Input: dimensioned drawing with shaded views. Units: mm. Origin: part minimum x, y, z. Round coordinates to 2 decimals unless told otherwise and drop trailing zeros. Write each loop counter-clockwise with the first axis right and the second up, starting at its lowest first coordinate (ties: lowest second). Pieces come first, ordered by that corner, then holes. Notation, with made-up numbers: (33.5, 19) - (68.5, 19) arc R7 ccw to (68.5, 24) - close; hole circle Ø8 at (66, 82.5). An arc over 180 degrees is marked (long way). Write item = value, one per line. Start each with the question number.
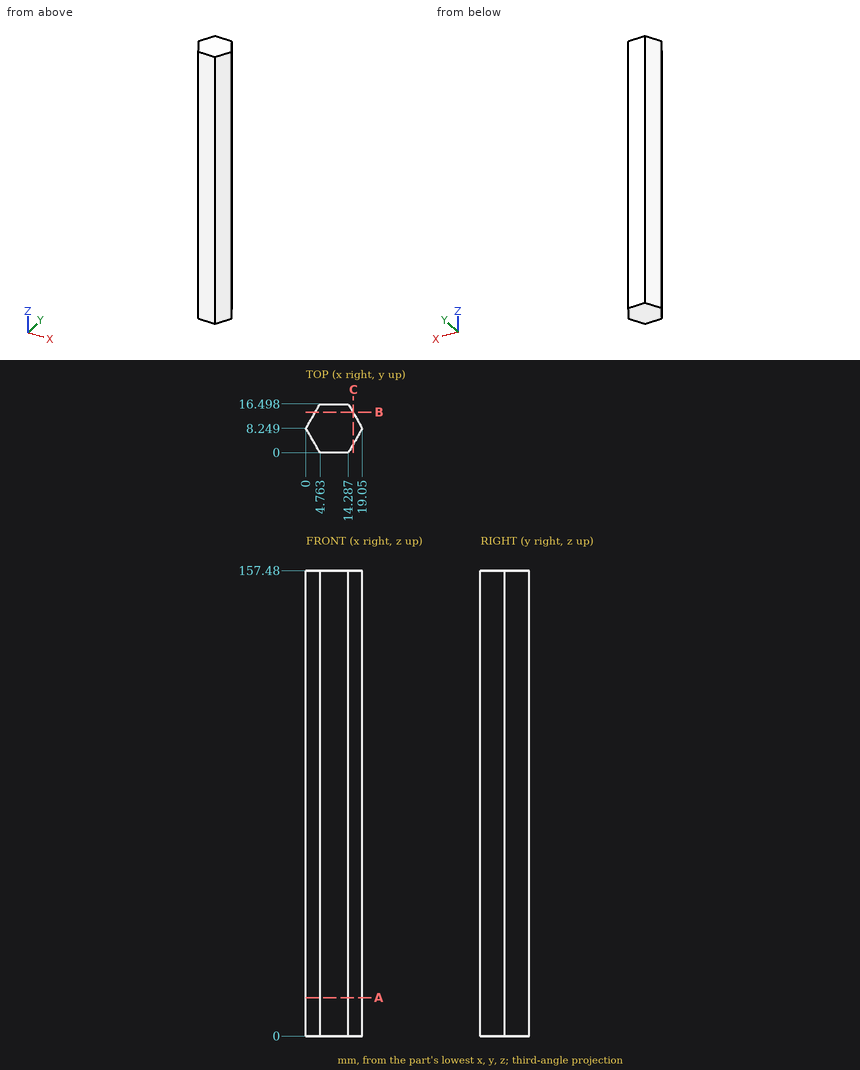
(1) Contact query for flat-ended pins moving along their axis: P1, Ø1.5, axis at y = 4, z = 103, coming from the +X side; P2, Ø1, axis at y = 10, z = 130, coming from the +X side; P3, Ø2, axis at x = 3.5, z = 86, coming from the -Y side (1 decimal). Output: stop coordinate, or through.
(2) Ray query, L1, parallel to Y at x = 4.75, z = 53.5 (1 decimal); L2, parallel to X at y = 14.5, z = 126; L3, parallel to X at y = 7, z = 48.5. Return the intervals inside material, ascending. Write a range as from..to.
(3) Section B-B (y = 13.75). Return the cut outline in (x, z).
(4) Section C-C (x = 16). Return the cut outline in (y, z), plus the area to 3 significant figures.
(5) Section A-A (z = 13). Return the cut outline in (x, y).
Solution:
q1.P1 = 17.03
q1.P2 = 18.33
q1.P3 = 0.5
q2.L1 = 0..16.5
q2.L2 = 3.61..15.44
q2.L3 = 0.72..18.33
q3.outline = (3.18, 0) - (15.87, 0) - (15.87, 157.48) - (3.18, 157.48) - close
q4.outline = (2.97, 0) - (13.53, 0) - (13.53, 157.48) - (2.97, 157.48) - close
q4.area = 1,660 mm^2
q5.outline = (0, 8.25) - (4.76, 0) - (14.29, 0) - (19.05, 8.25) - (14.29, 16.5) - (4.76, 16.5) - close
